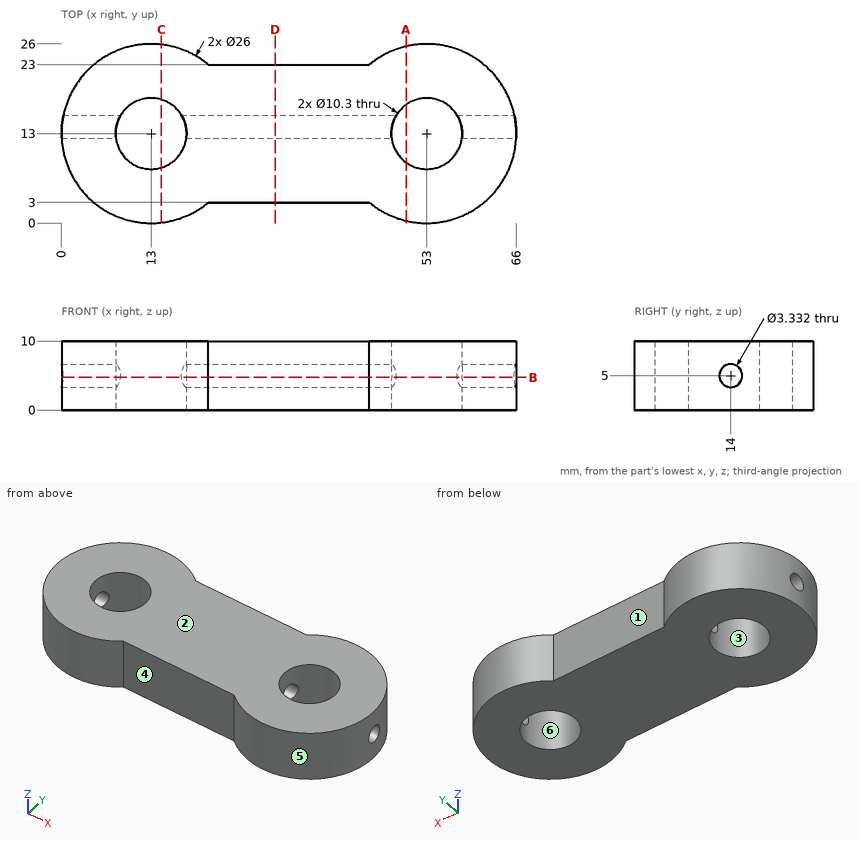
Input: dimensioned drawing with shaded views. Units: mm. Origin: part minimum x, y, z. A direction names the side the tool comes from. Coordinates: 2 decimals unless noted, no trailing zeros. Loops run counter-clockwise (first coordinate to the right, second up) from the corner with the lowest first, then second, coordinate; pieces in that order, holes last. Notation, with made-up numbers: (-9, -29.5) -> (22, -29.5) arc R11 ccw to (22, -21.5) -> close; hole circle Ø11 at (-15, 30.5). An arc over 180 degrees is marked (long way). Use a Markdown table: item, result. Add a question column.
(1) Section query A-A, the plane x = 50. Return loops of the section in (y, z).
(2) Mould query, pull axis Y, two halves, no side actions, for the marked faces 3, 4, 5 and 6. Classes: pulls with the +Y half, pulls with the -Y half, needs draft (parallel to the pull), parting line crosses it, or undercut.
(3) Access query for the marked faces 1 and 2. Directions: +Z, -Z, +X, -X, +Y, -Y. A direction counts if a zero-diameter tool reaches every point of the face in a straight line with its end or side. Return the directions, or none.
(4) Line query: line 1 along X through (y, z) = (15.75, 6); line 2 along X through (y, z) = (16.5, 7.25); line 3 along Y through (x, z) = (33.5, 9.25). Output: solid intervals per line, ascending.
(5) Section query D-D, the plane x = 31. Return loops of the section in (y, z).
(6) Section query C-C, the plane x = 14.5. Return loops of the section in (y, z).
(7) Pin query (flat end, axial travel): pin 1 Ø5 at (y, z) = (6.5, 3.5) entering from +X; pin 2 Ø6 at (x, z) = (47, 8) entering from -Y. Return the tip coordinate at first contact, or that it passes through.
(8) Section query B-B, the plane z = 4.75. Return loops of the section in (x, y), plus the area to 3 significant figures.
Answer:
| question | item | result |
|---|---|---|
| 1 | outline | (0.35, 0) -> (8.81, 0) -> (8.81, 10) -> (0.35, 10) -> close; (17.19, 0) -> (25.65, 0) -> (25.65, 10) -> (17.19, 10) -> close |
| 2 | face 3 | undercut |
| 2 | face 4 | pulls with the -Y half |
| 2 | face 5 | parting line crosses it |
| 2 | face 6 | undercut |
| 3 | face 1 | +Z, -Z, +Y |
| 3 | face 2 | +Z, +X, -X, +Y, -Y |
| 4 | line 1 | x = 0.29 to 8.65, 17.35 to 48.65, 57.35 to 65.71 |
| 4 | line 2 | x = 0.48 to 9.22, 16.78 to 49.22, 56.78 to 65.52 |
| 4 | line 3 | y = 3 to 23 |
| 5 | outline | (3, 0) -> (23, 0) -> (23, 10) -> (3, 10) -> close; hole circle Ø3.33 at (14, 5) |
| 6 | outline | (0.09, 0) -> (8.07, 0) -> (8.07, 10) -> (0.09, 10) -> close; (17.93, 0) -> (25.91, 0) -> (25.91, 10) -> (17.93, 10) -> close |
| 7 | pin 1 | stops at x = 65.37 |
| 7 | pin 2 | stops at y = 0.35 |
| 8 | outline | (0.02, 12.35) arc R13 ccw to (21.31, 3) -> (44.69, 3) arc R13 ccw to (65.98, 12.35) -> (58.11, 12.35) arc R5.15 cw to (47.89, 12.35) -> (18.11, 12.35) arc R5.15 cw to (7.89, 12.35) -> close; (0.27, 15.65) -> (8.58, 15.65) arc R5.15 cw to (17.42, 15.65) -> (48.58, 15.65) arc R5.15 cw to (57.42, 15.65) -> (65.73, 15.65) arc R13 ccw to (44.69, 23) -> (21.31, 23) arc R13 ccw to start |
| 8 | area | 1,080 mm^2 |
